from build123d import *

# Parameters (mm, degrees)
POCKET_DEPTH = 5.001


with BuildPart() as part:
    # Sketch → Revolution (revolve)
    with BuildSketch(Plane.YZ):
        Polygon((-14, 0), (-14, -1), (-2.8, -1), (-2.8, -5), (-2.3, -5), (-2.3, 0), align=None)
    revolve(axis=Axis((0, 0, 0), (0, 0, 1)))

    # Sketch001 (on Face6 of Revolution) → Pocket (cut, through all)
    with BuildSketch(Plane(origin=(0, 0, 0), x_dir=(0, -1, 0), z_dir=(0, 0, 1))):
        with BuildLine():
            Line((-13.9942845476, 0.4), (-3.4641016151, 0.5))
            ThreePointArc((-3.4641016151, -0.5), (3.5, 0), (-3.4641016151, 0.5))
            Line((-3.4641016151, -0.5), (-13.9942845476, -0.4))
            ThreePointArc((-13.9942845476, -0.4), (14, 0), (-13.9942845476, 0.4))
        make_face()
    extrude(amount=-POCKET_DEPTH, mode=Mode.SUBTRACT)


solid = part.part
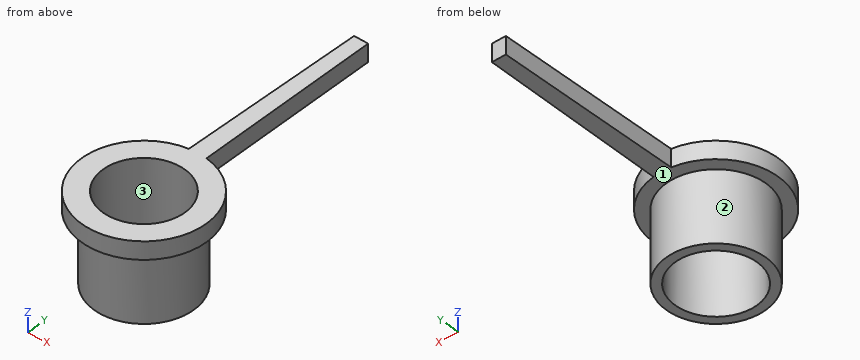
Part model, mm, in its own coordinate system. Face numbers are marked on the shaded views. Round coordinates to 2 decimals unless told otherwise and drop trailing zeros. Order: outer loops, then holes, each group sorted by start corner. A loop starts at its lowest first (then second) coordinate and runs counter-clockwise, first axis right, second up. Notation, with made-up numbers: (56, 27.25) -> (77, 27.25) arc R13 ccw to (77, 34.25) -> close; hole circle Ø8 at (70, -16). An arc over 180 degrees is marked (long way). Put each result on its own line as item: value.
Q1. Pin check, flat tips, straight feed: pin 1 Ø1 at (y, z) = (-1.5, -3) entering from -X; pin 2 Ø1.5 at (x, y) = (-1, 10.5) entering from -Z; pin 3 Ø1.5 at (x, y) = (-1.5, 5) entering from +Z. Stop position of each tip, or through.
From the geometry:
pin 1: stops at x = -2.62
pin 2: stops at z = -1
pin 3: passes through
Q2. Band-saw the part on B-B (x = 0). Give the cut face in (y, z), and give its area (3 significant figures).
From the geometry:
outline: (-3.5, -1) -> (-2.8, -1) -> (-2.8, -5) -> (-2.3, -5) -> (-2.3, 0) -> (-3.5, 0) -> close; (2.3, -5) -> (2.8, -5) -> (2.8, -1) -> (14, -1) -> (14, 0) -> (2.3, 0) -> close
area: 16.9 mm2
Q3. Wall check: line 1 (X direction, y = 0, z = -3.9); line 2 (X direction, y = -1.75, z = -2.1); line 3 (Y direction, x = -1.25, z = -4). Give the ranges that are in metal, low to high. Write a range as [from, to].
From the geometry:
line 1: x = [-2.8, -2.3], [2.3, 2.8]
line 2: x = [-2.19, -1.49], [1.49, 2.19]
line 3: y = [-2.51, -1.93], [1.93, 2.51]
Q4. Band-saw the part on A-A (y = 0). Give the cut face in (x, z), and give its area (3 significant figures).
From the geometry:
outline: (-3.5, -1) -> (-2.8, -1) -> (-2.8, -5) -> (-2.3, -5) -> (-2.3, 0) -> (-3.5, 0) -> close; (2.3, -5) -> (2.8, -5) -> (2.8, -1) -> (3.5, -1) -> (3.5, 0) -> (2.3, 0) -> close
area: 6.40 mm2
Q5. Pull direction Y, two halves, no side cores. Call the marked faces 1, 2 and 3: pulls with the +Y half, pulls with the -Y half, needs draft (parallel to the pull), parting line crosses it, or undercut.
From the geometry:
face 1: needs draft
face 2: parting line crosses it
face 3: undercut
Q6. Band-saw the part on C-C (z = -0.35). Give the cut face in (x, y).
From the geometry:
outline: (-0.5, 3.46) arc R3.5 ccw (long way) to (0.5, 3.46) -> (0.4, 13.99) arc R14 ccw to (-0.4, 13.99) -> close; hole circle Ø4.6 at (0, 0)
Q7. Band-saw the part on D-D (x = -2.5). Give the cut face in (y, z).
From the geometry:
outline: (-2.45, -1) -> (-1.26, -1) -> (-1.26, -5) -> (1.26, -5) -> (1.26, -1) -> (2.45, -1) -> (2.45, 0) -> (-2.45, 0) -> close
